Geometry check sheet. Reference: the model listing, model coordinates, mm. Face numbers are marked on the shaded views. A direction names the side the tool comes from. Round coordinates to 2 decimals unless told otherwise and drop trailing zeros. Loops run counter-clockwise (first coordinate to the right, second up) from the corner with the lowest first, then second, coordinate; pieces in that order, holes last. Notation, with made-up numbers: (11, -9.5) - (37, -9.5) arc R14 ccw to (37, 9.5) - close; hole circle Ø5 at (-38, 77). An arc over 180 degrees is marked (long way). Write item = value, one per line.
```python
from build123d import *

# Parameters (mm, degrees)
BOSS_EXTRUDE1_DEPTH      = 7.5
BOSS_EXTRUDE1_DEPTH_BACK = 7.5
SKETCH1_W                = 59
SKETCH1_H                = 48
SKETCH2_W                = 41
SKETCH2_H                = 4
CUT_EXTRUDE1_DEPTH       = 57.837487629
SKETCH3_W                = 59
SKETCH3_H                = 28
CUT_EXTRUDE2_DEPTH       = 4
SKETCH4_W                = 28
SKETCH4_H                = 11
CUT_EXTRUDE3_DEPTH       = 4


with BuildPart() as part:
    # Sketch1 → Boss-Extrude1 (new, two sides: drawn at the far end of the back side and taken through both)
    with BuildSketch(Plane(origin=(0, 0, 0), x_dir=(1, 0, 0), z_dir=(0, 1, 0)).offset(-BOSS_EXTRUDE1_DEPTH_BACK)):
        Rectangle(SKETCH1_W, SKETCH1_H)
    extrude(amount=BOSS_EXTRUDE1_DEPTH + BOSS_EXTRUDE1_DEPTH_BACK)

    # Sketch2 → Cut-Extrude1 (cut, through all)
    with BuildSketch(Plane.XY.offset(24)):
        Rectangle(SKETCH2_W, SKETCH2_H)
    extrude(amount=-CUT_EXTRUDE1_DEPTH, mode=Mode.SUBTRACT)

    # Sketch3 → Cut-Extrude2 (cut)
    with BuildSketch(Plane(origin=(0, 7.5, 0), x_dir=(1, 0, 0), z_dir=(0, 1, 0))):
        Rectangle(SKETCH3_W, SKETCH3_H)
    cut_extrude2 = extrude(amount=-CUT_EXTRUDE2_DEPTH, mode=Mode.SUBTRACT)

    # Sketch4 → Cut-Extrude3 (cut)
    with BuildSketch(Plane.ZY.offset(29.5)):
        with Locations((0, -2)):
            Rectangle(SKETCH4_W, SKETCH4_H)
    cut_extrude3 = extrude(amount=-CUT_EXTRUDE3_DEPTH, mode=Mode.SUBTRACT)

    # Mirror1: Cut-Extrude3 across plane
    add(cut_extrude3.mirror(Plane(origin=(0, 0, 0), x_dir=(0, 0, 1), z_dir=(1, 0, 0))), mode=Mode.SUBTRACT)

    # Mirror2: Cut-Extrude2 across plane
    add(cut_extrude2.mirror(Plane.ZX), mode=Mode.SUBTRACT)


solid = part.part
```
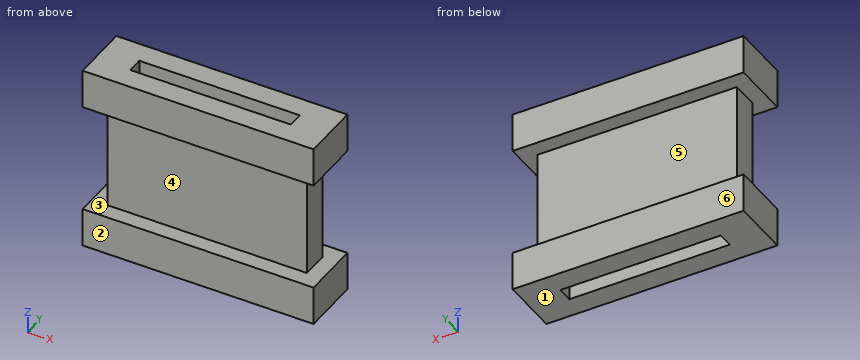
(1) Section check D-D (y = 5.25). Enter the section's corners in (x, z).
Answers follow:
outline = (-29.5, -24) - (29.5, -24) - (29.5, -14) - (-29.5, -14) - close; (-29.5, 14) - (29.5, 14) - (29.5, 24) - (-29.5, 24) - close
(2) Scan lines: L1, parallel to Y at x = -11, z = 15; L2, parallel to Y at x = 15, z = -7; L3, parallel to Z at x = -6.5, y = -5.5. Record each from-to range of solid material in increasing order. Write a range as [from, to].
Answers follow:
L1 = [-7.5, -2], [2, 7.5]
L2 = [-3.5, -2], [2, 3.5]
L3 = [-24, -14], [14, 24]
(3) Section check B-B (y = -1.25). Enter the section's corners in (x, z).
Answers follow:
outline = (-29.5, -24) - (-20.5, -24) - (-20.5, 24) - (-29.5, 24) - (-29.5, 14) - (-25.5, 14) - (-25.5, -14) - (-29.5, -14) - close; (20.5, -24) - (29.5, -24) - (29.5, -14) - (25.5, -14) - (25.5, 14) - (29.5, 14) - (29.5, 24) - (20.5, 24) - close
(4) Section check C-C (z = 12). Enter the section's corners in (x, y).
Answers follow:
outline = (-25.5, -3.5) - (25.5, -3.5) - (25.5, 3.5) - (-25.5, 3.5) - close; hole (-20.5, -2) - (20.5, -2) - (20.5, 2) - (-20.5, 2) - close
(5) Mould release check, pull along Z, two halves, no side actions. Record for the marked faces 1, 2 and 3: pulls with the +Z half, pulls with the -Z half, needs draft (parallel to the pull), parting line crosses it, or undercut.
Answers follow:
face_1 = pulls with the -Z half
face_2 = needs draft
face_3 = undercut
(6) Gauge pin test, flat ends, axial feed: pin 1 (2 mm diameter, centred on y = -1, z = 9.5, fed in from +X); pin 2 (8.5 mm diameter, centred on x = -9, z = 0.5, fed in from -Y); pin 3 (6 mm diameter, centred on y = -3.5, z = -9, fed in from -X). Record the tip position at first contact, or that the pin passes through.
Answers follow:
pin_1 = 25.5
pin_2 = -3.5
pin_3 = -25.5
(7) Section check A-A (x = 2.5). Enter the section's corners in (y, z), then the cut area to 3 significant figures.
Answers follow:
outline = (-7.5, -24) - (-2, -24) - (-2, 24) - (-7.5, 24) - (-7.5, 14) - (-3.5, 14) - (-3.5, -14) - (-7.5, -14) - close; (2, -24) - (7.5, -24) - (7.5, -14) - (3.5, -14) - (3.5, 14) - (7.5, 14) - (7.5, 24) - (2, 24) - close
area = 304 mm²
(8) Set-up check for the marked faces 4, 5 and 6: record each of +Z, -Z, +X, -X, +Y, -Y from which the full face is reachable in a straight line by a thin tool's end or side.
Answers follow:
face_4 = +X, -X, -Y
face_5 = +X, -X, +Y
face_6 = +Z, -Z, +X, -X, +Y
